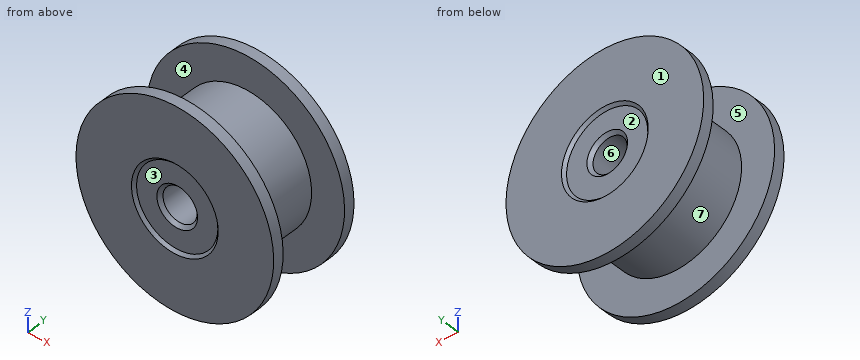
```python
from build123d import *

# Parameters (mm, degrees)
SKETCH1_R           = 6
BOSS_EXTRUDE1_DEPTH = 3.25
SKETCH2_R           = 9
BOSS_EXTRUDE2_DEPTH = 1
SKETCH4_R           = 4
CUT_EXTRUDE1_DEPTH  = 16.305227865
SKETCH7_R           = 4
SKETCH7_R_2         = 1.55
BOSS_EXTRUDE4_DEPTH = 4
CHAMFER2_SIZE       = 0.3


with BuildPart() as part:
    # Sketch1 → Boss-Extrude1 (new, symmetric)
    with BuildSketch(Plane(origin=(0, 0, 0), x_dir=(1, 0, 0), z_dir=(0, 1, 0))):
        with Locations(Location((0, 0, 0), (0, 0, 90))):
            Circle(SKETCH1_R)
    extrude(amount=BOSS_EXTRUDE1_DEPTH, both=True)

    # Sketch2 → Boss-Extrude2 (add)
    with BuildSketch(Plane(origin=(0, 3.25, 0), x_dir=(1, 0, 0), z_dir=(0, 1, 0))):
        with Locations(Location((0, 0, 0), (0, 0, 270))):
            Circle(SKETCH2_R)
    boss_extrude2 = extrude(amount=BOSS_EXTRUDE2_DEPTH)

    # Mirror3: Boss-Extrude2 across plane
    add(boss_extrude2.mirror(Plane.ZX))

    # Sketch4 → Cut-Extrude1 (cut, through all)
    with BuildSketch(Plane.XZ.offset(4.25)):
        with Locations(Location((0, 0, 0), (0, 0, 270))):
            Circle(SKETCH4_R)
    extrude(amount=-CUT_EXTRUDE1_DEPTH, mode=Mode.SUBTRACT)

    # Sketch7 → Boss-Extrude4 (add, symmetric)
    with BuildSketch(Plane(origin=(0, 0, 0), x_dir=(1, 0, 0), z_dir=(0, 1, 0))):
        with Locations(Location((0, 0, 0), (0, 0, 90))):
            Circle(SKETCH7_R)
        with Locations(Location((0, 0, 0), (0, 0, 270))):
            Circle(SKETCH7_R_2, mode=Mode.SUBTRACT)
    extrude(amount=BOSS_EXTRUDE4_DEPTH, both=True)

    # Chamfer2
    # the kernel refuses this chamfer: 0.3 mm, written as the material it adds along each edge
    with BuildSketch(Plane(origin=(0, 4, 0), x_dir=(0, 0, -1), z_dir=(1, 0, 0))) as chamfer2_piece_1_section:
        Polygon((4 - CHAMFER2_SIZE, 0), (4, CHAMFER2_SIZE), (4, 0), align=None)
    chamfer2_piece_1 = revolve(axis=Axis((0, 4, 0), (0, 1, 0)), mode=Mode.PRIVATE)
    chamfer2_piece_1 = split(chamfer2_piece_1, bisect_by=Plane(origin=(0, 4.25, 3.828198445), z_dir=(0, -1, 0)), keep=Keep.TOP, mode=Mode.PRIVATE)
    add(chamfer2_piece_1)
    with BuildSketch(Plane(origin=(0, -4, 0), x_dir=(0, 0, -1), z_dir=(1, 0, 0))) as chamfer2_piece_2_section:
        Polygon((4, -CHAMFER2_SIZE), (4 - CHAMFER2_SIZE, 0), (4, 0), align=None)
    chamfer2_piece_2 = revolve(axis=Axis((0, -4, 0), (0, 1, 0)), mode=Mode.PRIVATE)
    chamfer2_piece_2 = split(chamfer2_piece_2, bisect_by=Plane(origin=(0, -4.25, 3.828198445), z_dir=(0, 1, 0)), keep=Keep.TOP, mode=Mode.PRIVATE)
    add(chamfer2_piece_2)
    # the kernel refuses this chamfer: 0.3 mm, written as the material it takes off along each edge
    with BuildSketch(Plane(origin=(0, 4, 0), x_dir=(0, 0, 1), z_dir=(-1, 0, 0))) as chamfer2_2_piece_1:
        Polygon((1.55, -CHAMFER2_SIZE), (1.55 + CHAMFER2_SIZE, 0), (1.55, 0), align=None)
    revolve(axis=Axis((0, 4, 0), (0, 1, 0)), mode=Mode.SUBTRACT)
    with BuildSketch(Plane(origin=(0, -4, 0), x_dir=(0, 0, 1), z_dir=(-1, 0, 0))) as chamfer2_2_piece_2:
        Polygon((1.55 + CHAMFER2_SIZE, 0), (1.55, CHAMFER2_SIZE), (1.55, 0), align=None)
    revolve(axis=Axis((0, -4, 0), (0, 1, 0)), mode=Mode.SUBTRACT)


solid = part.part
```
Can you work these out from the model? Positions are in its coordinate system, mm. Face numbers are marked on the shaded views. A direction names the side the tool comes from. Round coordinates to 2 decimals unless told otherwise and drop trailing zeros. Loops run counter-clockwise (first coordinate to the right, second up) from the corner with the lowest first, then second, coordinate; pieces in that order, holes last. Notation, with made-up numbers: M 11.5,-6.75 L 34.5,-6.75 A16 cw 34.5,1.25 Z; hole C 40,23 d5. An arc over 180 degrees is marked long. Answer as a JSON object with one key per item and string values. Group by question number.
Q1. Imagine slicing it at B-B, the plane x = 0. Please give me the cut outline in (y, z), then the cut area to 3 significant figures.
Q2. Please list where these lines run through material, in increasing order: L1, parallel to Y at x = -2.5, z = -5.75; L2, parallel to X at y = -1, z = 0; L3, parallel to Z at x = -4.5, y = 1.75.
Q3. On a 3-axis mill with a long thin cutter (end or side, diameter ignored), from which of +Z, -Z, +X, -X, +Y, -Y can I reach the whole of each face in a straight line? I mean the marked faces 1, 2, 3 and 4. Say none if no direction works.
Q4. Imagine slicing it at A-A, the plane z = 0. Please give me the cut outline in (x, y), then the cut area to 3 significant figures.
Q5. Imagine slicing it at D-D, the plane z = -5.75. Please give me the cut outline in (x, y), then the cut area to 3 significant figures.
Q6. Will these pins go through, and if not, where does the flat tip stop? pin 1 (3 mm diameter, centred on x = 5, y = 2.5, fed in from +Z); pin 2 (5 mm diameter, centred on y = -0.5, z = 6, fed in from +X); pin 3 (1 mm diameter, centred on x = 7, y = -2, fed in from -Z); pin 4 (3 mm diameter, centred on x = -4.5, y = -1, fed in from +Z).
Q7. We'd pull the mould along X, two halves only. Please class the marked faces 5, 6 and 7: +X half, -X half, draft (parallel to the pull), parting line (faces both ways), or undercut.
Q8. Imagine slicing it at C-C, the plane y = -0.5. Please give me the cut outline in (x, z), then the cut area to 3 significant figures.
Findings:
{
 "1": {"outline": "M -4.25,-9 L -3.25,-9 L -3.25,-6 L 3.25,-6 L 3.25,-9 L 4.25,-9 L 4.25,-3.95 L 4,-3.7 L 4,-1.85 L 3.7,-1.55 L -3.7,-1.55 L -4,-1.85 L -4,-3.7 L -4.25,-3.95 Z; M -4.25,3.95 L -4,3.7 L -4,1.85 L -3.7,1.55 L 3.7,1.55 L 4,1.85 L 4,3.7 L 4.25,3.95 L 4.25,9 L 3.25,9 L 3.25,6 L -3.25,6 L -3.25,9 L -4.25,9 Z", "area": "85.2 mm2"},
 "2": {"L1": "y = -4.25 to -3.25, 3.25 to 4.25", "L2": "x = -6 to -1.55, 1.55 to 6", "L3": "z = -3.97 to 3.97"},
 "3": {"face 1": "+Z, -Z, +X, -X, +Y", "face 2": "+Y", "face 3": "-Y", "face 4": "none"},
 "4": {"outline": "M -9,-4.25 L -3.95,-4.25 L -3.7,-4 L -1.85,-4 L -1.55,-3.7 L -1.55,3.7 L -1.85,4 L -3.7,4 L -3.95,4.25 L -9,4.25 L -9,3.25 L -6,3.25 L -6,-3.25 L -9,-3.25 Z; M 1.55,-3.7 L 1.85,-4 L 3.7,-4 L 3.95,-4.25 L 9,-4.25 L 9,-3.25 L 6,-3.25 L 6,3.25 L 9,3.25 L 9,4.25 L 3.95,4.25 L 3.7,4 L 1.85,4 L 1.55,3.7 Z", "area": "85.2 mm2"},
 "5": {"outline": "M -6.92,-4.25 L 6.92,-4.25 L 6.92,-3.25 L 1.71,-3.25 L 1.71,3.25 L 6.92,3.25 L 6.92,4.25 L -6.92,4.25 L -6.92,3.25 L -1.71,3.25 L -1.71,-3.25 L -6.92,-3.25 Z", "area": "50.0 mm2"},
 "6": {"pin 1": "stops at z = 8.2", "pin 2": "stops at x = 4.87", "pin 3": "passes through", "pin 4": "stops at z = 5.2"},
 "7": {"face 5": "draft", "face 6": "undercut", "face 7": "parting line"},
 "8": {"outline": "C 0,0 d12; hole C 0,0 d3.1", "area": "106 mm2"}
}
